Could you check a few things on this model? Use its own coordinates, in mm. A direction names the side the tool comes from. Coordinates: 2 decimals unless noted, no trailing zeros. Write each loop counter-clockwise with the first axis right and the second up, starting at its lowest first coordinate (ties: lowest second). Pieces come first, ordered by that corner, then holes.
Item 1: Which directions (+Z, -Z, +X, -X, +Y, -Y) give clear straight access to the entire face, cutting with the end or side of a thin tool? Please do faces 5 (the flat face through (37, -50.3, 1)), 6 (the flat face through (0, -32, 18)).
Item 2: Thinking about a two-plate mould opening in Y: for faces 1 (the flat face through (1.48, -2.76, 65.31)), 2 (the flat face through (18, -65, 1)), 3 (the cylindrical face through (1.48, -57.74, 64.39)), 4 (the flat face through (3, -46, 22)), which applies, +Y half, -Y half, draft (parallel to the pull), parting line (faces both ways), or undercut?
Item 3: I want a section at A-A on y = -8.95. Please give me the cut outline in (x, z).
Item 4: I want a section at C-C on x = 54. Please give me the cut outline in (y, z), then the cut area to 3 significant figures.
Item 5: If I drill on probe 1 along Z at (x, y) = (0.8, -56.05); probe 2 along Z at (x, y) = (2, -32.5); probe 3 along Y at (x, z) = (1.85, 39), over which ranges is the centre line in solid material (lowest first)?
Item 6: I want a section at B-B on z = 15.45. Please give me the cut outline in (x, y).
Item 7: For P1, Ø1.5, axis at x = 38, z = 2, coming from the +Y side; P2, Ø1, axis at x = 57, y = -49, coming from the +Z side; P3, Ø8, axis at y = -45, z = 24.5, coming from the +X side, each with a flat end and sliding along its axis, tell me the tip position at first contact or that it passes through.
Item 8: I want a section at D-D on y = -32.5. Please give me the cut outline in (x, z).
from build123d import *

# Parameters (mm, degrees)
PAD_DEPTH       = 65
SKETCH001_R     = 19.05
SKETCH001_R_2   = 2.5
POCKET_DEPTH    = 3
POCKET001_DEPTH = 3


with BuildPart() as part:
    # Sketch → Pad (new body)
    with BuildSketch(Plane.XZ):
        Polygon((0, 0), (0, 68), (3, 68), (3, 3), (68, 3), (68, 0), align=None)
    extrude(amount=PAD_DEPTH)

    # Sketch001 (on Face1 of Pad) → Pocket (cut)
    with BuildSketch(Plane(origin=(0, 0, 0), x_dir=(0, 0, -1), z_dir=(-1, 0, 0))):
        with Locations((-39, 32.5)):
            Circle(SKETCH001_R)
        with Locations((-62.55, 56.05)):
            Circle(SKETCH001_R_2)
        with Locations((-62.55, 8.95)):
            Circle(SKETCH001_R_2)
        with Locations((-15.45, 8.95)):
            Circle(SKETCH001_R_2)
        with Locations((-15.45, 56.05)):
            Circle(SKETCH001_R_2)
        Polygon((-62.55, 0), (-68, 0), (-68, 5.45), align=None)
        Polygon((-68, 59.55), (-68, 65), (-62.55, 65), align=None)
    extrude(amount=-POCKET_DEPTH, mode=Mode.SUBTRACT)

    # Sketch002 (on Face7 of Pocket) → Pocket001 (cut)
    with BuildSketch(Plane(origin=(0, 0, 0), x_dir=(1, 0, 0), z_dir=(0, 0, -1))):
        Polygon((62.55, 65), (68, 65), (68, 59.55), align=None)
        Polygon((62.55, 0), (68, 0), (68, 5.45), align=None)
        with BuildLine():
            ThreePointArc((16.15, 54.6), (14, 52.45), (16.15, 50.3))
            Line((16.15, 50.3), (57.85, 50.3))
            ThreePointArc((57.85, 50.3), (60, 52.45), (57.85, 54.6))
            Line((16.15, 54.6), (57.85, 54.6))
        make_face()
        with BuildLine():
            ThreePointArc((16.15, 14.6), (14, 12.45), (16.15, 10.3))
            Line((16.15, 10.3), (57.85, 10.3))
            ThreePointArc((57.85, 10.3), (60, 12.45), (57.85, 14.6))
            Line((16.15, 14.6), (57.85, 14.6))
        make_face()
    extrude(amount=-POCKET001_DEPTH, mode=Mode.SUBTRACT)


solid = part.part
Response values:
1. face 5: +Z, -Z
1. face 6: +Z, -Z, -X, +Y, -Y
2. face 1: +Y half
2. face 2: -Y half
2. face 3: undercut
2. face 4: draft
3. outline: (0, 0) - (68, 0) - (68, 3) - (3, 3) - (3, 12.95) - (0, 12.95) - close; (0, 17.95) - (3, 17.95) - (3, 60.05) - (0, 60.05) - close; (0, 65.05) - (3, 65.05) - (3, 68) - (0, 68) - close
4. outline: (-65, 0) - (-54.6, 0) - (-54.6, 3) - (-65, 3) - close; (-50.3, 0) - (-14.6, 0) - (-14.6, 3) - (-50.3, 3) - close; (-10.3, 0) - (0, 0) - (0, 3) - (-10.3, 3) - close
4. area: 169 mm2
5. probe 1: z = 0 to 12.95, 17.95 to 60.05, 65.05 to 68
5. probe 2: z = 0 to 19.95, 58.05 to 68
5. probe 3: y = -65 to -51.55, -13.45 to 0
6. outline: (0, -65) - (3, -65) - (3, -58.55) - (0, -58.55) - close; (0, -53.55) - (3, -53.55) - (3, -11.45) - (0, -11.45) - close; (0, -6.45) - (3, -6.45) - (3, 0) - (0, 0) - close
7. P1: stops at y = 0
7. P2: stops at z = 3
7. P3: stops at x = 3
8. outline: (0, 0) - (68, 0) - (68, 3) - (3, 3) - (3, 19.95) - (0, 19.95) - close; (0, 58.05) - (3, 58.05) - (3, 68) - (0, 68) - close
